```python
from build123d import *

# Parameters (mm, degrees)
SKETCH_1_W          = 30
SKETCH_1_H          = 20
EXTRUDE_1_DEPTH     = 20
CUT_EXTRUDE_1_DEPTH = 20
SKETCH_10_W         = 32.252295377
SKETCH_10_H         = 15.179180951
CUT_EXTRUDE_2_DEPTH = 25


with BuildPart() as part:
    # 草圖1 → 填料-伸長1 (new body)
    with BuildSketch(Plane(origin=(0, 0, 0), x_dir=(1, 0, 0), z_dir=(0, 1, 0))):
        Rectangle(SKETCH_1_W, SKETCH_1_H)
    extrude(amount=EXTRUDE_1_DEPTH)

    # 草圖6 → 除料-伸長1 (cut)
    with BuildSketch(Plane(origin=(3.947368421, 11.842105263, -11.842105263), x_dir=(0.973328527, -0.162221421, 0.162221421), z_dir=(-0.229415734, -0.688247202, 0.688247202))):
        Polygon((0, 0), (-20.538761547, 0), (-20.538761547, 12.535207186), (11.71353383, 14.625633738), (12.268136792, -0.263322726), align=None)
    extrude(amount=-CUT_EXTRUDE_1_DEPTH, mode=Mode.SUBTRACT)

    # 草圖10 → 除料-伸長2 (cut)
    with BuildSketch(Plane(origin=(-3.947368421, 11.842105263, 11.842105263), x_dir=(0.973328527, 0.162221421, 0.162221421), z_dir=(-0.229415734, 0.688247202, 0.688247202))):
        with Locations((3.943334428, 7.114500239)):
            Rectangle(SKETCH_10_W, SKETCH_10_H)
    extrude(amount=CUT_EXTRUDE_2_DEPTH, mode=Mode.SUBTRACT)


solid = part.part
```
The model under review builds one solid part; all positions refer to its coordinate system, in mm. Coordinates: 2 decimals unless noted, no trailing zeros. Order: outer loops, then holes, each group sorted by start corner. A loop starts at its lowest first (then second) coordinate and runs counter-clockwise, first axis right, second up. Notation, with made-up numbers: (-7, 63) -> (19, 63) arc R16 cw to (19, 70) -> close; hole circle Ø8 at (70.25, 65). An arc over 180 degrees is marked (long way). Answer in a Markdown table with one row per item. Add a question column.
Item 1: We need section B-B on z = -8.5. Write out the cut boundary in (x, y).
Item 2: Clearance check with a flat-ended pin moving along its axis: pin 1 (4 mm diameter, centred on x = -10.5, y = 14, fed in from +Z). State where the tip first meets the part, or that it passes through.
Item 3: Mouldability with a two-part tool opening along Y and no side actions: class faces 1 (the flat face through (0, 20, 0)), 2 (the flat face through (0, 0, 0)), 3 (the flat face through (15, 10, 0)) as +Y half, -Y half, draft (parallel to the pull), parting line (faces both ways), or undercut.
Item 4: We need section A-A on y = 16.25. Write out the cut boundary in (x, z), plus the area to 3 significant figures.
Item 5: We need section C-C on x = -9. Write out the cut boundary in (y, z), plus the area to 3 significant figures.
Item 6: We need section D-D on z = 5. Write out the cut boundary in (x, y), plus the area to 4 significant figures.
Item 7: To check wall thickness, follow probe 1 along Y at (x, z) = (-12.5, 3.5); probe 2 along Z at (x, y) = (-9, 18.5); probe 3 along Y at (x, z) = (11, -9). State the ranges of each line that lie inside material, in increasing order.
Final values:
| question | item | result |
|---|---|---|
| 1 | outline | (-15, 0) -> (15, 0) -> (15, 11.5) -> (-10.5, 20) -> (-15, 20) -> close |
| 2 | pin 1 | stops at z = 9.61 |
| 3 | face 1 | +Y half |
| 3 | face 2 | -Y half |
| 3 | face 3 | draft |
| 4 | outline | (-15, -10) -> (-3.75, -10) -> (15, -3.75) -> (15, 10) -> (3.75, 10) -> (-15, 3.75) -> close |
| 4 | area | 483 mm2 |
| 5 | outline | (0, -10) -> (18, -10) -> (20, -8) -> (20, 2) -> (12, 10) -> (0, 10) -> close |
| 5 | area | 366 mm2 |
| 6 | outline | (-15, 0) -> (15, 0) -> (15, 20) -> (0, 20) -> (-15, 15) -> close |
| 6 | area | 562.5 mm2 |
| 7 | probe 1 | y = 0 to 17.33 |
| 7 | probe 2 | z = -9.5 to 3.5 |
| 7 | probe 3 | y = 0 to 12.33 |
